Could you check a few things on this model? Use its own coordinates, in mm. A direction names the side the tool comes from. Round coordinates to 2 decimals unless told otherwise and drop trailing zeros. Write each loop counter-clockwise with the first axis right and the second up, starting at its lowest first coordinate (ties: lowest second). Pieces come first, ordered by that corner, then holes. Notation, with made-up numbers: (34, 61) - (85, 61) arc R14 cw to (85, 72) - close; hole circle Ø8 at (84, -17). An arc over 180 degrees is marked (long way). Put each result on its own line as item: value.
from build123d import *

# Parameters (mm, degrees)
SKETCH1_R             = 13
BOSS_EXTRUDE1_DEPTH   = 25
BOSS_EXTRUDE2_DEPTH   = 7.5
BOSS_EXTRUDE2_2_DEPTH = 7.5
BOSS_EXTRUDE3_DEPTH   = 15
SKETCH5_R             = 3
CUT_EXTRUDE1_DEPTH    = 40.389084782
SKETCH6_R             = 4.45
CUT_EXTRUDE2_DEPTH    = 3
SKETCH7_R             = 4
CUT_EXTRUDE3_DEPTH    = 7.5
BOSS_EXTRUDE6_REACH   = 57.809
SKETCH10_R            = 1.6
CUT_EXTRUDE4_DEPTH    = 56.808932723
SKETCH11_R            = 3.1
CUT_EXTRUDE5_DEPTH    = 48.070587643
SKETCH12_W            = 50
SKETCH12_H            = 50
CUT_EXTRUDE8_DEPTH    = 54.659969844


with BuildPart() as part:
    # Sketch1 → Boss-Extrude1 (new body)
    with BuildSketch(Plane.XY):
        Circle(SKETCH1_R)
    extrude(amount=-BOSS_EXTRUDE1_DEPTH)

    # Sketch2 → Cut-Revolve1 (revolve, cut)
    with BuildSketch(Plane(origin=(0, 0, 0), x_dir=(0, 0, -1), z_dir=(1, 0, 0)), mode=Mode.PRIVATE) as cut_revolve1_sk:
        Polygon((0, 0), (0, 7.6), (11.5, 9.5), (14, 10.6), (25, 11), (25, 0), align=None)
    revolve(cut_revolve1_sk.sketch.rotate(Axis((0, 0, -25), (0, 0, 1)), 90), axis=Axis((0, 0, -25), (0, 0, 1)), mode=Mode.SUBTRACT)



with BuildPart() as body_2:
    # Sketch3 → Boss-Extrude2 (new, symmetric)
    with BuildSketch(Plane(origin=(0, 0, 0), x_dir=(1, 0, 0), z_dir=(0, 1, 0))):
        with BuildLine():
            Line((-13, 25), (-13, 10))
            Line((-13, 10), (-15, 10))
            ThreePointArc((-15, 10), (-22.5, 17.5), (-15, 25))
            Line((-15, 25), (-13, 25))
        make_face()
    extrude(amount=BOSS_EXTRUDE2_DEPTH, both=True)


with BuildPart() as body_3:
    # Sketch3 → Boss-Extrude2 2 (new, symmetric)
    with BuildSketch(Plane(origin=(0, 0, 0), x_dir=(1, 0, 0), z_dir=(0, 1, 0))):
        with BuildLine():
            Line((13, 25), (15, 25))
            ThreePointArc((15, 25), (22.5, 17.5), (15, 10))
            Line((15, 10), (13, 10))
            Line((13, 10), (13, 25))
        make_face()
    extrude(amount=BOSS_EXTRUDE2_2_DEPTH, both=True)


with BuildPart() as part_1:
    add(part.part)

    add(body_2.part)  # Boss-Extrude3 merges body 2

    add(body_3.part)  # Boss-Extrude3 merges body 3
    # Sketch4 → Boss-Extrude3 (add)
    with BuildSketch(Plane(origin=(0, 0, -25), x_dir=(-1, 0, 0), z_dir=(0, 0, -1))):
        with BuildLine():
            Line((-13, 7.5), (-13, -7.5))
            Line((-13, -7.5), (-8.04673847, -7.5))
            ThreePointArc((-8.04673847, -7.5), (-11, 0), (-8.04673847, 7.5))
            Line((-8.04673847, 7.5), (-13, 7.5))
        make_face()
        with BuildLine():
            Line((13, 7.5), (13, -7.5))
            Line((13, -7.5), (8.04673847, -7.5))
            ThreePointArc((8.04673847, -7.5), (11, 0), (8.04673847, 7.5))
            Line((8.04673847, 7.5), (13, 7.5))
        make_face()
    extrude(amount=-BOSS_EXTRUDE3_DEPTH)

    # Sketch5 → Cut-Extrude1 (cut, through all)
    with BuildSketch(Plane(origin=(0, 7.5, 0), x_dir=(1, 0, 0), z_dir=(0, 1, 0))):
        with Locations(Location((16.9, 17.5, 0), (0, 0, 270))):
            Circle(SKETCH5_R)
        with Locations(Location((-16.9, 17.5, 0), (0, 0, 270))):
            Circle(SKETCH5_R)
    extrude(amount=-CUT_EXTRUDE1_DEPTH, mode=Mode.SUBTRACT)

    # Sketch6 → Cut-Extrude2 (cut)
    with BuildSketch(Plane(origin=(0, 7.5, 0), x_dir=(1, 0, 0), z_dir=(0, 1, 0))):
        with Locations(Location((-16.9, 17.5, 0), (0, 0, 270))):
            Circle(SKETCH6_R)
        with Locations(Location((16.9, 17.5, 0), (0, 0, 270))):
            Circle(SKETCH6_R)
    extrude(amount=-CUT_EXTRUDE2_DEPTH, mode=Mode.SUBTRACT)

    # Sketch7 → Cut-Extrude3 (cut)
    with BuildSketch(Plane.XZ.offset(7.5)):
        with Locations(Location((-16.9, -17.5, 0), (0, 0, 270))):
            Circle(SKETCH7_R)
        with Locations(Location((16.9, -17.5, 0), (0, 0, 270))):
            Circle(SKETCH7_R)
    extrude(amount=-CUT_EXTRUDE3_DEPTH, mode=Mode.SUBTRACT)

    # Sketch9 → Boss-Extrude6 (add, up to next)
    with BuildSketch(Plane(origin=(0, 24.373180657, -34.808509373), x_dir=(1, 0, 0), z_dir=(0, 0.5735764363510444, -0.819152044288993)), mode=Mode.PRIVATE) as boss_extrude6_sk1:
        with BuildLine():
            Line((-10.62, 5.324042616), (10.62, 5.324042616))
            Line((10.62, 5.324042616), (10.62, -0.669893629))
            ThreePointArc((10.62, -0.669893629), (7.308881484, -3.260182231), (3.4, -4.807355917))
            Line((3.4, -4.807355917), (3.4, -5.665957384))
            ThreePointArc((3.4, -5.665957384), (2.814213562, -7.080170946), (1.4, -7.665957384))
            Line((1.4, -7.665957384), (-1.4, -7.665957384))
            ThreePointArc((-1.4, -7.665957384), (-2.814213562, -7.080170946), (-3.4, -5.665957384))
            Line((-3.4, -5.665957384), (-3.4, -4.807355917))
            ThreePointArc((-3.4, -4.807355917), (-7.308881484, -3.260182231), (-10.62, -0.669893629))
            Line((-10.62, -0.669893629), (-10.62, 5.324042616))
        make_face()
    boss_extrude6_tool1 = extrude(boss_extrude6_sk1.sketch, amount=-BOSS_EXTRUDE6_REACH, mode=Mode.PRIVATE) - part_1.part
    add(boss_extrude6_tool1.solids().sort_by_distance((0, 24.258264, -34.888975))[0])

    # Sketch10 → Cut-Extrude4 (cut, through all)
    with BuildSketch(Plane(origin=(0, 24.373180657, -34.808509373), x_dir=(-1, 0, 0), z_dir=(0, 0.5735764363510444, -0.819152044288993))):
        with Locations(Location((-4, -0.484042616, 0), (0, 0, 90))):
            Circle(SKETCH10_R)
        with Locations(Location((4, -0.484042616, 0), (0, 0, 90))):
            Circle(SKETCH10_R)
    extrude(amount=-CUT_EXTRUDE4_DEPTH, mode=Mode.SUBTRACT)

    # Sketch11 → Cut-Extrude5 (cut, through all)
    with BuildSketch(Plane(origin=(0, 18.637416293, -26.61698893), x_dir=(1, 0, 0), z_dir=(0, 0.5735764363510444, -0.819152044288993))):
        with Locations(Location((4, 0.484042616, 0), (0, 0, 270))):
            Circle(SKETCH11_R)
        with Locations(Location((-4, 0.484042616, 0), (0, 0, 270))):
            Circle(SKETCH11_R)
    extrude(amount=-CUT_EXTRUDE5_DEPTH, mode=Mode.SUBTRACT)

    # Sketch12 → Cut-Extrude8 (cut, through all)
    with BuildSketch(Plane(origin=(0, 0, 0), x_dir=(1, 0, 0), z_dir=(0, 1, 0))):
        with Locations((0, 14.017641389)):
            Rectangle(SKETCH12_W, SKETCH12_H)
    extrude(amount=-CUT_EXTRUDE8_DEPTH, mode=Mode.SUBTRACT)


solid = part_1.part
(1) I'm going to push flat-ended pins straight in: pin 1 (9.5 mm diameter, centred on x = 18, z = -14, fed in from +Y); pin 2 (5 mm diameter, centred on y = 17.5, z = -22.5, fed in from -X); pin 3 (1.5 mm diameter, centred on y = 27, z = -33, fed in from +X); pin 4 (5 mm diameter, centred on x = -16.9, z = -17.5, fed in from -Y). Where does each tip first touch, or does it pass through?
Values found:
pin 1: stops at y = 7.5
pin 2: stops at x = -10.62
pin 3: stops at x = 8.58
pin 4: passes through
(2) Imagine slicing it at C-C, the plane z = -29.5. Give the number of separate pieces and of enclosed holes in the cut face, then the cut area to 3 significant figures.
Values found:
separate pieces: 1
enclosed holes: 2
area: 236 mm^2
(3) Imagine slicing it at A-A, the plane x = -16.9. List the corners of the cut face in (y, z) for me.
Values found:
outline: (0, -24.76) - (7.5, -24.76) - (7.5, -21.95) - (4.5, -21.95) - (4.5, -20.5) - (0, -20.5) - close; (0, -14.5) - (4.5, -14.5) - (4.5, -13.05) - (7.5, -13.05) - (7.5, -10.24) - (0, -10.24) - close
(4) For faces 4 (the face through (10.62, 16, -27)), 5 (the face through (-3.4, 20.5, -20.2)), 6 (the face through (-12.5, 7.5, -15.9)), 7 (the face through (13, 5, -10)), 8 (the face through (9.2, 4.1, -12.8)), which set-ups out of +Z, -Z, +X, -X, +Y, -Y let a thin tool reach every point of the face, with its end or its side?
Values found:
face 4: +Z, -Z, +X, +Y
face 5: +Z, -X, +Y
face 6: +Z, -Z, -X, +Y
face 7: +Z, +X, +Y
face 8: -Z, -Y
(5) If we mould it in two halves opening along Z, with no side actions, what happens to faces 1 (the face through (-3.93, 19.84, -31.965)), 2 (the face through (2.83, 21.41, -18.26)), 3 (the face through (0.2, 10.8, -19.6))? For each: pulls with the +Z half, pulls with the -Z half, needs draft (parallel to the pull), parting line crosses it, or undercut.
Values found:
face 1: undercut
face 2: pulls with the +Z half
face 3: pulls with the -Z half
(6) Please list where these lines run through material, in increasing order: probe 1 along X at (y, z) = (11, -19); probe 2 along X at (y, z) = (1.6, -17.5); probe 3 along X at (y, z) = (2, -17). Write a range as from..to.
Values found:
probe 1: x = -10.62..-6.76, -1.24..1.24, 6.76..10.62
probe 2: x = -22.5..-19.9, -13.9..-10.61, 10.61..13.9, 19.9..22.5
probe 3: x = -22.48..-19.86, -13.94..-10.52, 10.52..13.94, 19.86..22.48
